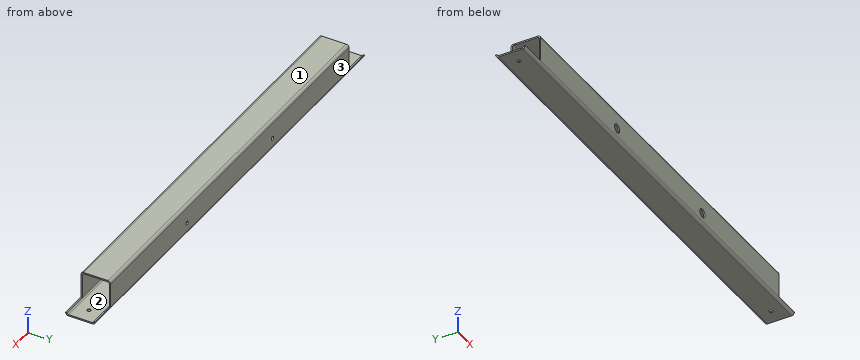
```python
from build123d import *

# Parameters (mm, degrees)
SHS_C450_AS_50X50X2_3_SHS_C450_1_DEPTH = 788
CUT_EXTRUDE1_DEPTH                     = 396.583113896
CUT_EXTRUDE1_DEPTH_BACK                = 396.583113896
SKETCH20_W                             = 45
SKETCH20_H                             = 45
SKETCH21_R                             = 3.25
CUT_EXTRUDE2_DEPTH                     = 10
SKETCH22_R                             = 3.25
CUT_EXTRUDE3_DEPTH                     = 10
SKETCH23_R                             = 7.5
CUT_EXTRUDE4_DEPTH                     = 10


with BuildPart() as part:
    # Sketch19 → Shs c450 as 50X50X2.3 SHS C450(1) (new body)
    with BuildSketch(Plane.YZ.offset(-394)):
        with BuildLine():
            Line((-20.4, -25), (20.4, -25))
            ThreePointArc((20.4, -25), (23.652691193, -23.652691193), (25, -20.4))
            Line((25, -20.4), (25, 20.4))
            ThreePointArc((25, 20.4), (23.652691193, 23.652691193), (20.4, 25))
            Line((20.4, 25), (-20.4, 25))
            ThreePointArc((-20.4, 25), (-23.652691193, 23.652691193), (-25, 20.4))
            Line((-25, 20.4), (-25, -20.4))
            ThreePointArc((-25, -20.4), (-23.652691193, -23.652691193), (-20.4, -25))
        make_face()
        with BuildLine():
            Line((-20.4, 22.7), (20.4, 22.7))
            ThreePointArc((20.4, 22.7), (22.026345597, 22.026345597), (22.7, 20.4))
            Line((22.7, 20.4), (22.7, -20.4))
            ThreePointArc((22.7, -20.4), (22.026345597, -22.026345597), (20.4, -22.7))
            Line((20.4, -22.7), (-20.4, -22.7))
            ThreePointArc((-20.4, -22.7), (-22.026345597, -22.026345597), (-22.7, -20.4))
            Line((-22.7, -20.4), (-22.7, 20.4))
            ThreePointArc((-22.7, 20.4), (-22.026345597, 22.026345597), (-20.4, 22.7))
        make_face(mode=Mode.SUBTRACT)
    extrude(amount=SHS_C450_AS_50X50X2_3_SHS_C450_1_DEPTH)

    # Sketch20 → Cut-Extrude1 (cut, two sides: drawn at the far end of the back side and taken through both)
    with BuildSketch(Plane(origin=(0, 0, 0), x_dir=(1, 0, 0), z_dir=(0, 1, 0)).offset(-CUT_EXTRUDE1_DEPTH_BACK)):
        with Locations((-371.5, -2.5)):
            Rectangle(SKETCH20_W, SKETCH20_H)
        with Locations((371.5, -2.5)):
            Rectangle(SKETCH20_W, SKETCH20_H)
    extrude(amount=CUT_EXTRUDE1_DEPTH + CUT_EXTRUDE1_DEPTH_BACK, mode=Mode.SUBTRACT)

    # Sketch21 → Cut-Extrude2 (cut)
    with BuildSketch(Plane(origin=(0, 0, -25), x_dir=(-1, 0, 0), z_dir=(0, 0, -1))):
        with Locations((-369, 0)):
            Circle(SKETCH21_R)
        with Locations((369, 0)):
            Circle(SKETCH21_R)
    extrude(amount=-CUT_EXTRUDE2_DEPTH, mode=Mode.SUBTRACT)

    # Sketch22 → Cut-Extrude3 (cut)
    with BuildSketch(Plane(origin=(0, 25, 0), x_dir=(1, 0, 0), z_dir=(0, 1, 0))):
        with Locations(Location((-125, 6, 0), (0, 0, 180))):
            Circle(SKETCH22_R)
        with Locations(Location((125, 6, 0), (0, 0, 180))):
            Circle(SKETCH22_R)
    extrude(amount=-CUT_EXTRUDE3_DEPTH, mode=Mode.SUBTRACT)

    # Sketch23 → Cut-Extrude4 (cut)
    with BuildSketch(Plane.XZ.offset(25)):
        with Locations((-125, -6)):
            Circle(SKETCH23_R)
        with Locations((125, -6)):
            Circle(SKETCH23_R)
    extrude(amount=-CUT_EXTRUDE4_DEPTH, mode=Mode.SUBTRACT)


solid = part.part
```
Check sheet for the modelled part. Datum: model origin and axes. Units: mm. Face numbers are marked on the shaded views. Coordinates: 2 decimals unless noted, no trailing zeros. Loops run counter-clockwise (first coordinate to the right, second up) from the corner with the lowest first, then second, coordinate; pieces in that order, holes last. Notation, with made-up numbers: M 44.5,-31 L 66.5,-31 A23 cw 66.5,-2 Z; hole C -22.5,-28.5 d1. An arc over 180 degrees is marked long. Answer as a JSON object with one key per item and string values.
1. Sectioned sample at B-B on z = 10. Record the cut outline in (x, y).
Outcome:
{"outline": "M -349,-25 L 349,-25 L 349,-22.7 L -349,-22.7 Z; M -349,22.7 L 349,22.7 L 349,25 L -349,25 Z"}
2. Scan lines: L1, parallel to Y at x = 4, z = -1; L2, parallel to Y at x = -276, z = 22. Record each from-to range of solid material in increasing order. Write a range as from..to.
Outcome:
{"L1": "-25..-22.7, 22.7..25", "L2": "-24.71..-22.05, 22.05..24.71"}
3. Sectioned sample at A-A on x = -341.5. Record the cut outline in (y, z).
Outcome:
{"outline": "M -25,-20.4 A4.6 ccw -20.4,-25 L 20.4,-25 A4.6 ccw 25,-20.4 L 25,20.4 A4.6 ccw 20.4,25 L -20.4,25 A4.6 ccw -25,20.4 Z; hole M -22.7,-20.4 A2.3 ccw -20.4,-22.7 L 20.4,-22.7 A2.3 ccw 22.7,-20.4 L 22.7,20.4 A2.3 ccw 20.4,22.7 L -20.4,22.7 A2.3 ccw -22.7,20.4 Z"}
4. Sectioned sample at C-C on y = 13.5. Record the cut outline in (x, z), and give its area (3 significant figures).
Outcome:
{"outline": "M -394,-25 L 394,-25 L 394,-22.7 L -394,-22.7 Z; M -349,22.7 L 349,22.7 L 349,25 L -349,25 Z", "area": "3,420 mm²"}
5. Release check for a two-part mould opening along Z. For the marked faces 1, 2 and 3 record: pulls with the +Z half, pulls with the -Z half, needs draft (parallel to the pull), parting line crosses it, or undercut.
Outcome:
{"face 1": "pulls with the +Z half", "face 2": "undercut", "face 3": "needs draft"}
6. Depth check by flat-ended pin: P1, Ø7.5, axis at x = -125, z = -6, coming from the -Y side; P2, Ø0.7, axis at x = -369.5, y = 23.5, coming from the +Z side. Enter the tip coordinate at first touch or a pass-through.
Outcome:
{"P1": "y = 22.7", "P2": "z = -20"}
